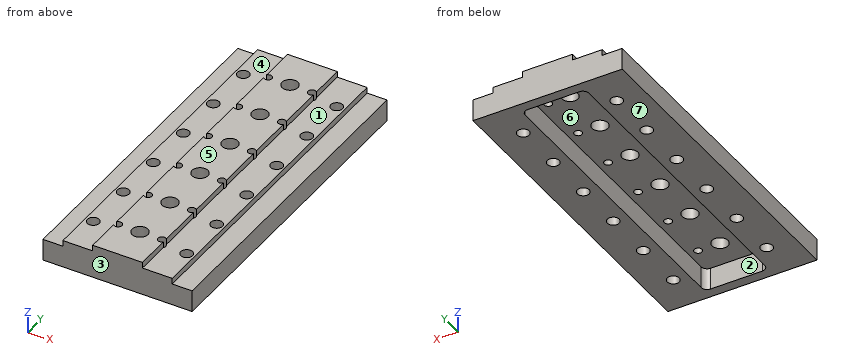
```python
from build123d import *

# Parameters (mm, degrees)
F1_DEPTH  = 165
F3_D      = 6
F4_D      = 3.9
F5_D      = 8
F6_W      = 32
F6_H      = 155
F7_DEPTH  = 11
F8_R      = 3
F10_W     = 10
F10_H     = 165
F11_DEPTH = 3
F9_W      = 10
F9_H      = 165
F12_DEPTH = 3


with BuildPart() as f1:
    # F0 (on Front) → F1 (new body)
    with BuildSketch(Plane.XZ):
        Polygon((0, 14), (0, 0), (75, 0), (75, 14), (50, 14), (50, 17), (25, 17), (25, 14), align=None)
    extrude(amount=F1_DEPTH)

    # F3 (through all)
    with Locations(Plane(origin=(0, 0, 0), x_dir=(1, 0, 0), z_dir=(0, 0, -1))):
        with Locations((14, 146), (14, 120.6), (14, 95.2), (14, 69.8), (14, 44.4), (14, 19), (61, 146), (61, 120.6), (61, 95.2), (61, 69.8), (61, 44.4), (61, 19)):
            Hole(F3_D / 2)

    # F4 (through all)
    with Locations(Plane(origin=(0, 0, 0), x_dir=(1, 0, 0), z_dir=(0, 0, -1))):
        with Locations((26.5, 146), (26.5, 120.6), (26.5, 95.2), (26.5, 69.8), (26.5, 44.4), (26.5, 19), (48.5, 19), (48.5, 44.4), (48.5, 69.8), (48.5, 95.2), (48.5, 120.6), (48.5, 146)):
            Hole(F4_D / 2)

    # F5 (through all)
    with Locations(Plane(origin=(0, 0, 0), x_dir=(1, 0, 0), z_dir=(0, 0, -1))):
        with Locations((37.5, 146), (37.5, 120.6), (37.5, 95.2), (37.5, 69.8), (37.5, 44.4), (37.5, 19)):
            Hole(F5_D / 2)

    # F6 (on face) → F7 (cut)
    with BuildSketch(Plane(origin=(0, 0, 0), x_dir=(1, 0, 0), z_dir=(0, 0, -1))):
        with Locations((37.5, 82.5)):
            Rectangle(F6_W, F6_H)
    extrude(amount=-F7_DEPTH, mode=Mode.SUBTRACT)

    # F8
    f8_edges = [f1.edges().sort_by_distance(p)[0] for p in [
        (21.5, -160, 5.5),
        (53.5, -160, 5.5),
        (21.5, -5, 5.5),
        (53.5, -5, 5.5),
    ]]
    fillet(f8_edges, radius=F8_R)

    # F10 (on face) → F11 (cut)
    with BuildSketch(Plane.XY.offset(14)):
        with Locations((5, -82.5)):
            Rectangle(F10_W, F10_H)
    extrude(amount=-F11_DEPTH, mode=Mode.SUBTRACT)

    # F9 (on face) → F12 (cut)
    with BuildSketch(Plane.XY.offset(14)):
        with Locations((70, -82.5)):
            Rectangle(F9_W, F9_H)
    extrude(amount=-F12_DEPTH, mode=Mode.SUBTRACT)


solid = f1.part
```
Geometry: final body of the model. Coordinates: model frame, mm. Face numbers are marked on the shaded views. A direction names the side the tool comes from. Coordinates: 2 decimals unless noted, no trailing zeros. Order: outer loops, then holes, each group sorted by start corner. A loop starts at its lowest first (then second) coordinate and runs counter-clockwise, first axis right, second up. Notation, with made-up numbers: M 22,20 L 65,20 A22 ccw 65,49 Z; hole C 68,49 d5. An arc over 180 degrees is marked long. Answer as CSV lines item,"result".
Q1. Section D-D on x = 31. Return the cut outline in (y, z).
Answers:
outline,"M -165,0 L -160,0 L -160,11 L -5,11 L -5,0 L 0,0 L 0,17 L -165,17 Z"
Q2. Section B-B on z = 4.5. Count the separate pieces of the cut face and the enclosed holes in it, and give its area (3 significant figures).
Answers:
separate pieces,"1"
enclosed holes,"13"
area,"7,080 mm^2"
Q3. Section A-A on x = 61. Return the cut outline in (y, z), and give its area (3 significant figures).
Answers:
outline,"M -165,0 L -149,0 L -149,14 L -165,14 Z; M -143,0 L -123.6,0 L -123.6,14 L -143,14 Z; M -117.6,0 L -98.2,0 L -98.2,14 L -117.6,14 Z; M -92.2,0 L -72.8,0 L -72.8,14 L -92.2,14 Z; M -66.8,0 L -47.4,0 L -47.4,14 L -66.8,14 Z; M -41.4,0 L -22,0 L -22,14 L -41.4,14 Z; M -16,0 L 0,0 L 0,14 L -16,14 Z"
area,"1,810 mm^2"
Q4. Draft query along X for the marked faces 6 and 7. Return one class per face: pulls with the +X half, pulls with the -X half, needs draft (parallel to the pull), parting line crosses it, or undercut.
Answers:
face 6,"undercut"
face 7,"needs draft"
Q5. Set-up query: the marked faces 1, 2, 3, 4 and 5. Return all of +Z, -Z, +X, -X, +Y, -Y with unobstructed straight access to the full face (end or side cutting, diameter ignored); none if empty.
Answers:
face 1,"+Z, +X, +Y, -Y"
face 2,"-Z"
face 3,"+Z, -Z, +X, -X, -Y"
face 4,"+Z, -X, +Y, -Y"
face 5,"+Z, +X, -X, +Y, -Y"
Q6. First-contact query: P1, Ø5, axis at x = 14, y = -19, coming from the -Z side; P2, Ø3.5, axis at y = -106.5, z = 15, coming from the -X side; P3, Ø1, axis at x = 65, y = -104, coming from the +Z side; P4, Ø1.5, axis at y = -106.5, z = 15.5, coming from the +X side. Flat tips, straight axial feed; report the tip coordinate or a pass-through.
Answers:
P1,"passes through"
P2,"stops at x = 10"
P3,"stops at z = 14"
P4,"stops at x = 50"
Q7. Section C-C on y = -109. Return the cut outline in (x, z).
Answers:
outline,"M 0,0 L 21.5,0 L 21.5,11 L 53.5,11 L 53.5,0 L 75,0 L 75,11 L 65,11 L 65,14 L 50,14 L 50,17 L 25,17 L 25,14 L 10,14 L 10,11 L 0,11 Z"
Q8. Line query: probe 1 along X at (y, z) = (-120.6, 7); probe 2 along X at (y, z) = (-152.5, 3.25); probe 3 along Y at (x, z) = (44.5, 7). Output: solid intervals per line, ascending. Write a range as [from, to].
Answers:
probe 1,"x = [0, 11], [17, 21.5], [53.5, 58], [64, 75]"
probe 2,"x = [0, 21.5], [53.5, 75]"
probe 3,"y = [-165, -160], [-5, 0]"
